Design review of the part shown in the three views and the two pictorial views. Dimensions are in mm from the part's minimum x, y and z. Give positions to 0.01 mm unless a question says otherwise; leave off trailing zeros. Order: outer loops, then holes, each group sorted by start corner. A loop starts at its lowest first (then second) coordinate and runs counter-clockwise, first axis right, second up. Notation, with made-up numbers: (13.25, -23.5) - (46.25, -23.5) arc R29 cw to (46.25, -0.5) - close; hole circle Ø1 at (41, -11). An arc over 180 degrees is marked (long way). Write each question's results on one line, items separated by ' | '. Start each with the question number.
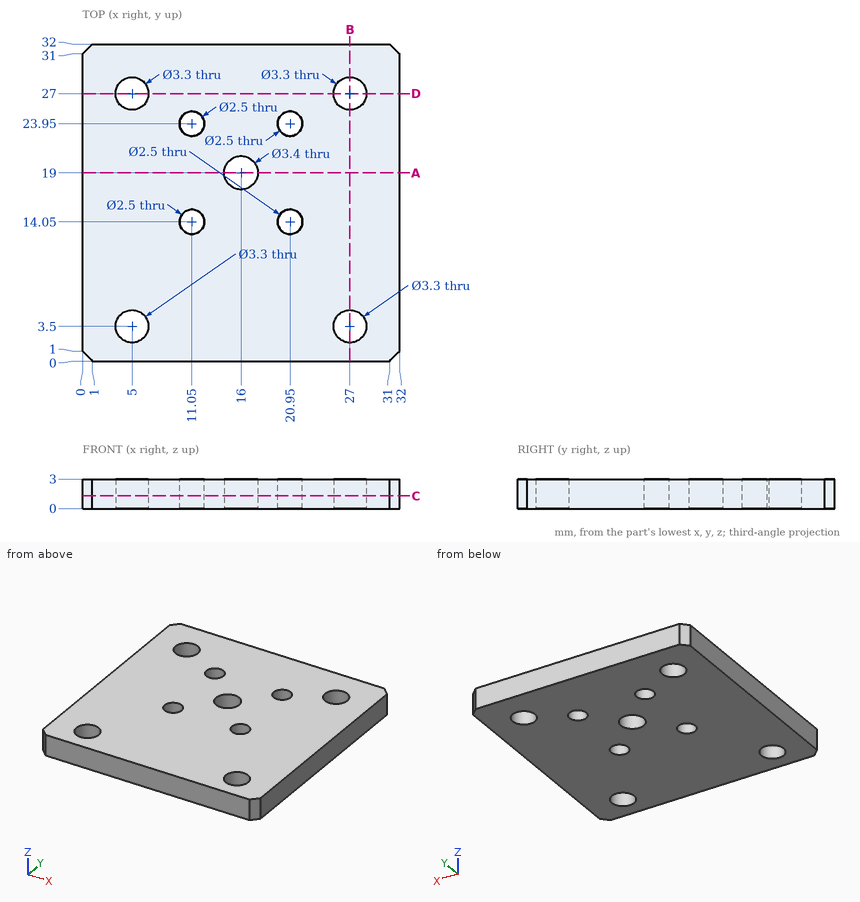
Q1. Add section B-B (x = 27). Give the boundary of the cut face in (y, z), plus the area to 3 significant figures.
Q2. Add section A-A (y = 19). Give the boundary of the cut face in (x, z), plus the area to 3 significant figures.
Q3. Insertion check: pin 1 Ø1.5 at (x, y) = (19.5, 14) entering from -Z. The pin has a flat end and moves straight along its axis. Give the tip position at first contact, or say it passes through.
Q4. Add section C-C (z = 1.3). Give the number of separate pieces and of enclosed holes in the cut face, plus the area to 3 significant figures.
Q5. For line 1 (Y direction, x = 27, z = 1.35); line 2 (Y direction, x = 21, z = 2.65); line 3 (X direction, y = 24.5, z = 1.1), list the stretches that pass through material, from the lowest coordinate up. Write a range as [from, to].
Q6. Add section D-D (y = 27). Give the boundary of the cut face in (x, z), plus the area to 3 significant figures.
Verdict:
1) outline: (0, 0) - (1.85, 0) - (1.85, 3) - (0, 3) - close; (5.15, 0) - (25.35, 0) - (25.35, 3) - (5.15, 3) - close; (28.65, 0) - (32, 0) - (32, 3) - (28.65, 3) - close | area: 76.2 mm2
2) outline: (0, 0) - (14.3, 0) - (14.3, 3) - (0, 3) - close; (17.7, 0) - (32, 0) - (32, 3) - (17.7, 3) - close | area: 85.8 mm2
3) pin 1: stops at z = 0
4) separate pieces: 1 | enclosed holes: 9 | area: 959 mm2
5) line 1: y = [0, 1.85], [5.15, 25.35], [28.65, 32] | line 2: y = [0, 12.8], [15.3, 22.7], [25.2, 32] | line 3: x = [0, 9.93], [12.17, 19.83], [22.07, 32]
6) outline: (0, 0) - (3.35, 0) - (3.35, 3) - (0, 3) - close; (6.65, 0) - (25.35, 0) - (25.35, 3) - (6.65, 3) - close; (28.65, 0) - (32, 0) - (32, 3) - (28.65, 3) - close | area: 76.2 mm2
